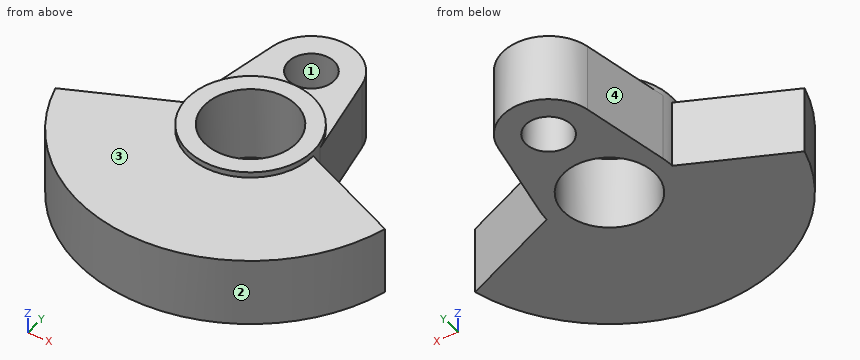
from build123d import *

# Parameters (mm, degrees)
BOSS_EXTRUDE1_DEPTH   = 3
SKETCH1_R             = 2
BOSS_EXTRUDE1_2_DEPTH = 3
BOSS_EXTRUDE2_START   = 3.5
SKETCH1_4_R           = 5.5
SKETCH1_4_R_2         = 4
BOSS_EXTRUDE2_DEPTH   = 6.5


with BuildPart() as part:
    # Sketch1 → Boss-Extrude1 (new, symmetric)
    with BuildSketch(Plane.XY):
        with BuildLine():
            Line((-5.5, 0), (-14.456832295, -4))
            ThreePointArc((-14.456832295, -4), (0, -15), (14.456832295, -4))
            Line((14.456832295, -4), (5.5, 0))
            ThreePointArc((5.5, 0), (0, -5.5), (-5.5, 0))
        make_face()
    extrude(amount=BOSS_EXTRUDE1_DEPTH, both=True)



with BuildPart() as body_2:
    # Sketch1 → Boss-Extrude1 2 (new, symmetric)
    with BuildSketch(Plane.XY):
        with BuildLine():
            Line((-3.929058411, 8.75), (-5.402455316, 1.03125))
            ThreePointArc((-5.402455316, 1.03125), (0, 5.5), (5.402455316, 1.03125))
            Line((5.402455316, 1.03125), (3.929058411, 8.75))
            ThreePointArc((3.929058411, 8.75), (0, 12), (-3.929058411, 8.75))
        make_face()
        with Locations((0, 8)):
            Circle(SKETCH1_R, mode=Mode.SUBTRACT)
    extrude(amount=BOSS_EXTRUDE1_2_DEPTH, both=True)


with BuildPart() as part_1:
    add(part.part)

    add(body_2.part)  # Boss-Extrude2 merges body 2
    # Sketch1<4> → Boss-Extrude2 (add)
    with BuildSketch(Plane.XY.offset(BOSS_EXTRUDE2_START)):
        Circle(SKETCH1_4_R)
        with Locations(Location((0, 0, 0), (0, 0, 180))):
            Circle(SKETCH1_4_R_2, mode=Mode.SUBTRACT)
    extrude(amount=-BOSS_EXTRUDE2_DEPTH)


solid = part_1.part
For this review, take the finished solid that the model builds, in its own axes (mm). Face numbers are marked on the shaded views. Coordinates: 2 decimals unless noted, no trailing zeros. Order: outer loops, then holes, each group sorted by start corner. A loop starts at its lowest first (then second) coordinate and runs counter-clockwise, first axis right, second up. Notation, with made-up numbers: (-5, 12) - (4, 12) arc R29 ccw to (4, 34) - close; hole circle Ø11 at (62, 39). An arc over 180 degrees is marked (long way). Answer as CSV lines item,"result". Start each with the question number.
1) Draft analysis for pull direction Y (two halves, no side actions). For the marked faces 1, 2, 3 and 4, state which applies: +Y half, -Y half, draft (parallel to the pull), parting line (faces both ways), or undercut.
2) Insertion check: P1, Ø8, axis at x = 7, y = -4, coming from the +Z side; P2, Ø1.5, axis at x = -3, z = -1, coming from the -Y side; P3, Ø3, axis at x = 2.5, z = 1, coming from the -Y side; P4, Ø5.5, axis at x = -1.5, y = 8.5, coming from the +Z side. Each pin has a flat end and moves straight along its axis. Give the tip position at first contact, or say it passes through.
3) Add section D-D (x = -3.5). State the section outline as (y, z) points, then the cut area to 3 significant figures.
4) Add section B-B (z = -1.75). State the section outline as (x, y) points.
5) Add section A-A (x = 0). State the section outline as (y, z) points, then the cut area to 3 significant figures.
6) Add section C-C (y = 7.5). State the section outline as (x, z) points, then the cut area to 3 significant figures.
7) To check wall thickness, follow line 1 along Y through (x, z) = (0, -1.5); line 2 along Y through (x, z) = (-1.25, 0.5); line 3 along Z through (x, y) = (12, -6.5). State the ranges of each line that lie inside material, in increasing order. Write a range as [from, to].
Result:
1,face 1,"undercut"
1,face 2,"-Y half"
1,face 3,"draft"
1,face 4,"+Y half"
2,P1,"z = 3.5"
2,P2,"y = -14.83"
2,P3,"y = -14.97"
2,P4,"z = 3"
3,outline,"(-14.59, -3) - (-1.94, -3) - (-1.94, 3.5) - (-4.24, 3.5) - (-4.24, 3) - (-14.59, 3) - close; (1.94, -3) - (9.94, -3) - (9.94, 3) - (4.24, 3) - (4.24, 3.5) - (1.94, 3.5) - close"
3,area,"126 mm^2"
4,outline,"(-14.46, -4) arc R15 ccw to (14.46, -4) - (5.5, 0) arc R5.5 ccw to (5.4, 1.03) - (3.93, 8.75) arc R4 ccw to (-3.93, 8.75) - (-5.4, 1.03) arc R5.5 ccw to (-5.5, 0) - close; hole circle Ø8 at (0, 0); hole circle Ø4 at (0, 8)"
5,outline,"(-15, -3) - (-4, -3) - (-4, 3.5) - (-5.5, 3.5) - (-5.5, 3) - (-15, 3) - close; (4, -3) - (6, -3) - (6, 3) - (5.5, 3) - (5.5, 3.5) - (4, 3.5) - close; (10, -3) - (12, -3) - (12, 3) - (10, 3) - close"
5,area,"91.5 mm^2"
6,outline,"(-4.17, -3) - (-1.94, -3) - (-1.94, 3) - (-4.17, 3) - close; (1.94, -3) - (4.17, -3) - (4.17, 3) - (1.94, 3) - close"
6,area,"26.8 mm^2"
7,line 1,"[-15, -4], [4, 6], [10, 12]"
7,line 2,"[-14.95, -3.8], [3.8, 6.44], [9.56, 11.8]"
7,line 3,"[-3, 3]"
